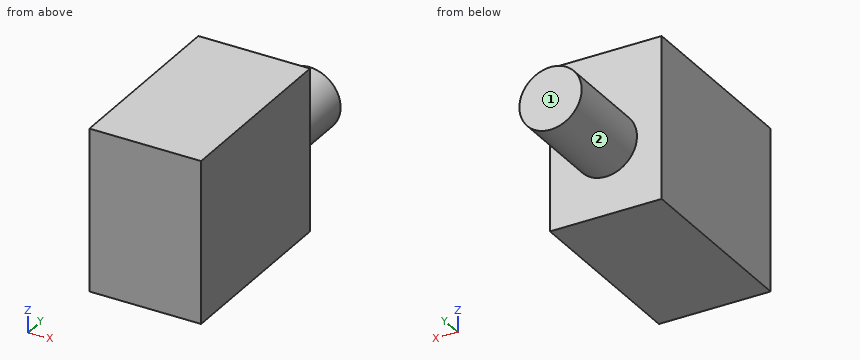
from build123d import *

# Parameters (mm, degrees)
F0_W     = 30
F0_H     = 50
F1_DEPTH = 1
F2_W     = 2
F2_H     = 2
F2_W_2   = 26
F2_H_2   = 46
F3_DEPTH = 40
F5_W     = 30
F5_H     = 50
F6_DEPTH = 2.54
F4_R     = 8.368495
F8_DEPTH = 25.4


with BuildPart() as f1:
    # F0 (on Top) → F1 (new body)
    with BuildSketch(Plane.XY):
        Rectangle(F0_W, F0_H)
    extrude(amount=F1_DEPTH)

    # F2 (on face) → F3 (join)
    with BuildSketch(Plane.XY.offset(1)):
        with Locations((-14, 24)):
            Rectangle(F2_W, F2_H)
        with Locations((0, 24)):
            Rectangle(F2_W_2, F2_H)
        with Locations((-14, 0)):
            Rectangle(F2_W, F2_H_2)
        with Locations((14, 24)):
            Rectangle(F2_W, F2_H)
        with Locations((-14, -24)):
            Rectangle(F2_W, F2_H)
        with Locations((0, -24)):
            Rectangle(F2_W_2, F2_H)
        with Locations((14, 0)):
            Rectangle(F2_W, F2_H_2)
        with Locations((14, -24)):
            Rectangle(F2_W, F2_H)
    extrude(amount=F3_DEPTH)

    # F5 (on face) → F6 (join)
    with BuildSketch(Plane.XY.offset(41)):
        Rectangle(F5_W, F5_H)
    extrude(amount=F6_DEPTH)

    # F4 (on face) → F8 (join)
    with BuildSketch(Plane(origin=(0, 25, 0), x_dir=(-1, 0, 0), z_dir=(0, 1, 0))):
        with Locations((0, 18.638214)):
            Circle(F4_R)
    extrude(amount=F8_DEPTH)


solid = f1.part
Source: CAD feature listing. Evaluate the final solid. Frame: model axes, mm. Face numbers are marked on the shaded views. A direction names the side the tool comes from. Round coordinates to 2 decimals unless told otherwise and drop trailing zeros. Write each loop counter-clockwise with the first axis right and the second up, starting at its lowest first coordinate (ties: lowest second). Pieces come first, ordered by that corner, then holes. Notation, with made-up numbers: M 23,41.5 L 71,41.5 A15 ccw 71,51.5 Z; hole C -25,88.25 d9. An arc over 180 degrees is marked long. One line per item, written item: value. Start each with the question number.
Item 1: Set-up query: the marked faces 1 and 2. Return all of +Z, -Z, +X, -X, +Y, -Y with unobstructed straight access to the full face (end or side cutting, diameter ignored); none if empty.
Item 2: Section query C-C (z = 21). Return the cut outline in (x, y).
Item 3: Section query A-A (x = -9.25). Return the cut outline in (y, z).
Item 4: Ray query, L1, parallel to Y at x = -9.25, z = 14; L2, parallel to Z at x = 7.5, y = 19.5; L3, parallel to X at y = 13, z = 32. Return the intervals inside material, ascending. Write a range as from..to.
Item 5: Section query B-B (z = 28). Return the cut outline in (x, y), plus the area to 3 significant figures.
Item 6: Section query D-D (x = 0). Return the cut outline in (y, z), plus the area to 3 significant figures.
Result set:
1. face 1: +Z, -Z, +X, -X, +Y
1. face 2: +Y
2. outline: M -15,-25 L 15,-25 L 15,25 L 8.03,25 L 8.03,50.4 L -8.03,50.4 L -8.03,25 L -15,25 Z; hole M -13,-23 L 13,-23 L 13,23 L -13,23 Z
3. outline: M -25,0 L 25,0 L 25,43.54 L -25,43.54 Z; hole M -23,1 L 23,1 L 23,41 L -23,41 Z
4. L1: y = -25..-23, 23..25
4. L2: z = 0..1, 41..43.54
4. L3: x = -15..-13, 13..15
5. outline: M -15,-25 L 15,-25 L 15,25 L -15,25 Z; hole M -13,-23 L 13,-23 L 13,23 L -13,23 Z
5. area: 304 mm²
6. outline: M -25,0 L 25,0 L 25,10.27 L 50.4,10.27 L 50.4,27.01 L 25,27.01 L 25,43.54 L -25,43.54 Z; hole M -23,1 L 23,1 L 23,41 L -23,41 Z
6. area: 762 mm²
